The model under review builds one solid part; all positions refer to its coordinate system, in mm. Coordinates: 2 decimals unless noted, no trailing zeros. Order: outer loops, then holes, each group sorted by start corner. A loop starts at its lowest first (then second) coordinate and runs counter-clockwise, first axis right, second up.
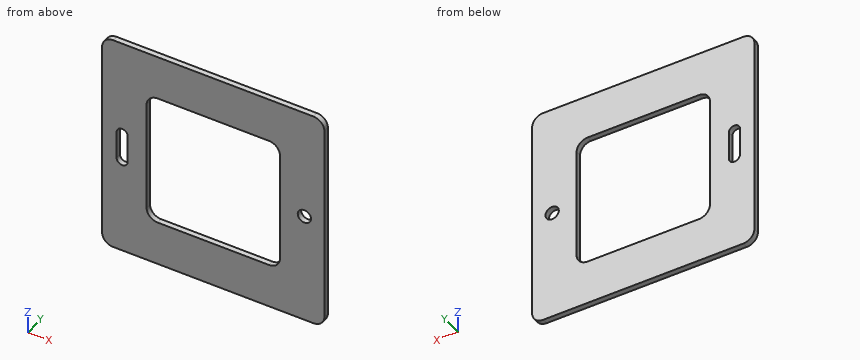
```python
from build123d import *

# Parameters (mm, degrees)
SKETCH1_W           = 200
SKETCH1_H           = 200
BOSS_EXTRUDE1_DEPTH = 5
SKETCH2_R           = 6
CUT_EXTRUDE1_DEPTH  = 12
REDONDEO1_R         = 10


with BuildPart() as part:
    # Sketch1 → Boss-Extrude1 (new body)
    with BuildSketch(Plane(origin=(0, 0, 0), x_dir=(1, 0, 0), z_dir=(0, 1, 0))):
        Rectangle(SKETCH1_W, SKETCH1_H)
        with BuildLine():
            Line((-50, -60), (50, -60))
            ThreePointArc((50, -60), (57.071067812, -57.071067812), (60, -50))
            Line((60, -50), (60, 50))
            ThreePointArc((60, 50), (57.071067812, 57.071067812), (50, 60))
            Line((50, 60), (-50, 60))
            ThreePointArc((-50, 60), (-57.071067812, 57.071067812), (-60, 50))
            Line((-60, 50), (-60, -50))
            ThreePointArc((-60, -50), (-57.071067812, -57.071067812), (-50, -60))
        make_face(mode=Mode.SUBTRACT)
    extrude(amount=BOSS_EXTRUDE1_DEPTH)

    # Sketch2 → Cut-Extrude1 (cut)
    with BuildSketch(Plane(origin=(0, 5, 0), x_dir=(1, 0, 0), z_dir=(0, 1, 0))):
        with Locations(Location((82, 0, 0), (0, 0, 270))):
            Circle(SKETCH2_R)
        with BuildLine():
            Line((-87, -12.5), (-87, 12.5))
            ThreePointArc((-87, 12.5), (-82, 17.5), (-77, 12.5))
            Line((-77, 12.5), (-77, -12.5))
            ThreePointArc((-77, -12.5), (-82, -17.5), (-87, -12.5))
        make_face()
    extrude(amount=-CUT_EXTRUDE1_DEPTH, mode=Mode.SUBTRACT)

    # Redondeo1
    redondeo1_edges = [part.edges().sort_by_distance(p)[0] for p in [
        (100, 2.5, 100),
        (-100, 2.5, 100),
        (-100, 2.5, -100),
        (100, 2.5, -100),
    ]]
    fillet(redondeo1_edges, radius=REDONDEO1_R)


solid = part.part
```
(1) We need section B-B, the plane z = -32. Write out the cut boundary in (x, y), and give its area (3 significant figures).
A:
outline: (-100, 0) - (-60, 0) - (-60, 5) - (-100, 5) - close; (60, 0) - (100, 0) - (100, 5) - (60, 5) - close
area: 400 mm2
(2) Wall thickness on probe 1 along X at (y, z) = (2.3, 0); probe 2 along Z at (x, y) = (2.5, 1.9); probe 3 along X at (y, z) = (4, 7.5): over which ranges is each line inside the solid? List them lowest first.
A:
probe 1: x = -100 to -87, -77 to -60, 60 to 76, 88 to 100
probe 2: z = -100 to -60, 60 to 100
probe 3: x = -100 to -87, -77 to -60, 60 to 100
(3) For pin 1 Ø6 at (x, z) = (-79.5, -54) entering from -Y, flat-tipped, find the tip position at first contact; note if it passes through.
A:
pin 1: stops at y = 0
(4) We need section C-C, the plane y = 3.55. Write out the cut boundary in (x, z), and give its area (3 significant figures).
A:
outline: (-100, -90) arc R10 ccw to (-90, -100) - (90, -100) arc R10 ccw to (100, -90) - (100, 90) arc R10 ccw to (90, 100) - (-90, 100) arc R10 ccw to (-100, 90) - close; hole (-87, -12.5) arc R5 ccw to (-77, -12.5) - (-77, 12.5) arc R5 ccw to (-87, 12.5) - close; hole (-60, -50) arc R10 ccw to (-50, -60) - (50, -60) arc R10 ccw to (60, -50) - (60, 50) arc R10 ccw to (50, 60) - (-50, 60) arc R10 ccw to (-60, 50) - close; hole circle Ø12 at (82, 0)
area: 25,200 mm2
(5) We need section A-A, the plane x = -82. Write out the cut boundary in (y, z), and give its area (3 significant figures).
A:
outline: (0, -100) - (5, -100) - (5, -17.5) - (0, -17.5) - close; (0, 17.5) - (5, 17.5) - (5, 100) - (0, 100) - close
area: 825 mm2
